```python
from build123d import *

# Parameters (mm, degrees)
SKETCH1_R           = 1.85
BOSS_EXTRUDE1_DEPTH = 3.175


with BuildPart() as part:
    # Sketch1 → Boss-Extrude1 (new body)
    with BuildSketch(Plane.XY):
        Polygon((156, 0), (0, 0), (0, 14.15), (-12.897437159, 26), (-72.0466, 26), (-72.0466, 48), (37.159, 48), (37.159, 60.975), (76.2722, 60.975), (76.2722, 32), (156, 32), align=None)
        with Locations((144, 8)):
            Circle(SKETCH1_R, mode=Mode.SUBTRACT)
        with Locations((144, 24)):
            Circle(SKETCH1_R, mode=Mode.SUBTRACT)
        with Locations((152, 16)):
            Circle(SKETCH1_R, mode=Mode.SUBTRACT)
        with Locations((136, 16)):
            Circle(SKETCH1_R, mode=Mode.SUBTRACT)
        with Locations((24, 16)):
            Circle(SKETCH1_R, mode=Mode.SUBTRACT)
        with Locations((16, 8)):
            Circle(SKETCH1_R, mode=Mode.SUBTRACT)
        with Locations((8, 16)):
            Circle(SKETCH1_R, mode=Mode.SUBTRACT)
        with Locations((16, 24)):
            Circle(SKETCH1_R, mode=Mode.SUBTRACT)
        with Locations((72, 16)):
            Circle(SKETCH1_R, mode=Mode.SUBTRACT)
    extrude(amount=BOSS_EXTRUDE1_DEPTH)


solid = part.part
```
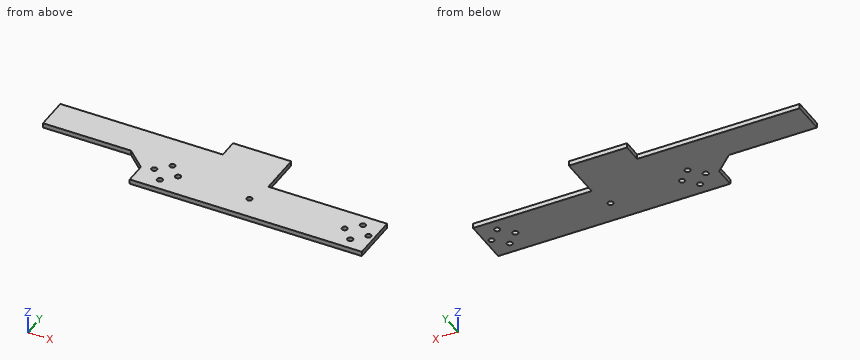
The listing builds one solid part. Answer for the finished solid, in the listing's coordinates (mm). Give positions to 0.01 mm unless a question says otherwise; leave off trailing zeros. Write each loop counter-clockwise with the first axis right and the second up, starting at its lowest first coordinate (ties: lowest second). Pieces come first, ordered by that corner, then holes. Notation, with made-up numbers: (89, 89.25) -> (125, 89.25) arc R18 cw to (125, 115.25) -> close; hole circle Ø5 at (55.5, 16). An arc over 180 degrees is marked (long way). Write item = value, one per line. Start each with the question number.
1) The part is cut by section B-B, the plane x = 126.5. Determine the outline of the cut face in (y, z) (3 decimals), and give its area (3 significant figures).
2) Straight lines are drawn through the part: line 1 along Y through (x, z) = (16, 1.15); line 2 along Y through (x, z) = (136, 0.95); line 3 along Y through (x, z) = (72, 1.8) (3 decimals). For each, find the intervals that lie inside material, in ascending order.
3) The part is cut by section C-C, the plane y = 45. Determine the outline of the cut face in (x, z) (3 decimals).
4) The part is cut by section A-A, the plane z = 2.35. Count the separate pieces of the cut face and the enclosed holes in it, and give its area (3 significant figures).
5) Each of these flat-tipped pins is pushed along its axis until it touches: pin 1 (1.6 mm diameter, centred on y = 54, z = 1.5, fed in from -X); pin 2 (5 mm diameter, centred on x = 16, y = 8, fed in from -Z); pin 3 (3.5 mm diameter, centred on x = 16, y = 24, fed in from -Z); pin 4 (1.6 mm diameter, centred on x = -32, z = 2, fed in from -Y). Where does it stop, or does it pass through?
Solutions:
q1.outline = (0, 0) -> (32, 0) -> (32, 3.175) -> (0, 3.175) -> close
q1.area = 102 mm²
q2.line_1 = 0 to 6.15, 9.85 to 22.15, 25.85 to 48
q2.line_2 = 0 to 14.15, 17.85 to 32
q2.line_3 = 0 to 14.15, 17.85 to 60.975
q3.outline = (-72.047, 0) -> (76.272, 0) -> (76.272, 3.175) -> (-72.047, 3.175) -> close
q4.separate_pieces = 1
q4.enclosed_holes = 9
q4.area = 8,280 mm²
q5.pin_1 = 37.16
q5.pin_2 = 0
q5.pin_3 = through
q5.pin_4 = 26
